Could you check a few things on this model? Use its own coordinates, in mm. A direction names the side the tool comes from. Give positions to 0.01 mm unless a question says otherwise; leave off trailing zeros. Write item = value, one per line.
from build123d import *

# Parameters (mm, degrees)
F0_W     = 12.5
F0_H     = 2.5
F2_W     = 5
F2_H     = 30
F3_DEPTH = 6


# Not quite as in the source:
# - a fillet or chamfer that OpenCascade refuses, or shapes differently, is made with other operations: its cross-section is extruded or revolved along the edge and cut away or added


with BuildPart() as f1:
    # F0 (on Front) → F1 (revolve)
    with BuildSketch(Plane.XZ):
        with BuildLine():
            Line((0, 2.5), (12.5, 2.5))
            add(Edge.make_bspline(
                [(8, 38), (7.0575290046, 36.0296102259), (4.9176459622, 31.9169764445), (8.8571855748, 23.8819266131), (11.7311727266, 17.2522437772), (5.0634432181, 9.5532988579), (9.6973287885, 5.0417102196), (12.5, 2.5)],
                knots=[0, 0, 0, 0, 0.1821407595, 0.3923850866, 0.5803644457, 0.7831417696, 1, 1, 1, 1], degree=3))
            Line((8, 38), (0, 38))
            Line((0, 38), (0, 2.5))
        make_face()
        with Locations((6.25, 1.25)):
            Rectangle(F0_W, F0_H)
        Polygon((10, 40), (10, 48), (8, 48), (8, 40), (0, 40), (0, 38), (8, 38), align=None)
    revolve(axis=Axis((0, 0, 44), (0, 0, -1)))

    # F2 (on face) → F3 (cut)
    with BuildSketch(Plane.XY.offset(48)):
        Rectangle(F2_W, F2_H)
    extrude(amount=-F3_DEPTH, mode=Mode.SUBTRACT)

    # F4: chamfer of 5 on 1 edges, made by hand


with BuildPart() as f4_tool2:
    # F4_s3 → F4_t4 (revolve)
    with BuildSketch(Plane.XZ):
        Polygon((8, 45), (3, 40), (8, 40), align=None)
    revolve(axis=Axis((0, 0, 40), (0, 0, -1)))

    split(bisect_by=Plane.YZ.offset(2.5), keep=Keep.TOP)


with BuildPart() as f1_1:
    add(f1.part)

    # F4_t1: union F4_tool2
    add(f4_tool2.part)


with BuildPart() as f4_tool7:
    # F4_s8 → F4_t9 (revolve)
    with BuildSketch(Plane.XZ):
        Polygon((8, 45), (3, 40), (8, 40), align=None)
    revolve(axis=Axis((0, 0, 40), (0, 0, -1)))

    split(bisect_by=Plane.XY.offset(42), keep=Keep.BOTTOM)


with BuildPart() as f1_2:
    add(f1_1.part)

    # F4_t6: union F4_tool7
    add(f4_tool7.part)


with BuildPart() as f4_tool12:
    # F4_s13 → F4_t14 (revolve)
    with BuildSketch(Plane.XZ):
        Polygon((8, 45), (3, 40), (8, 40), align=None)
    revolve(axis=Axis((0, 0, 40), (0, 0, -1)))

    split(bisect_by=Plane.YZ.offset(-2.5), keep=Keep.BOTTOM)


with BuildPart() as f1_3:
    add(f1_2.part)

    # F4_t11: union F4_tool12
    add(f4_tool12.part)


solid = f1_3.part
1. Thinking about a two-plate mould opening in Y: for faces 5 (the face through (0, -7, 42)), 6 (the face through (8, 0, 46)), 7 (the face through (11.923, -3.755, 1.268)), which applies, pulls with the +Y half, pulls with the -Y half, needs draft (parallel to the pull), parting line crosses it, or undercut?
Filled sheet:
face_5 = needs draft
face_6 = undercut
face_7 = parting line crosses it
2. For pin 1 (6 mm diameter, centred on y = 7, z = 44, fed in from +X); pin 2 (2.5 mm diameter, centred on x = 1, y = 7.5, fed in from +Z); pin 3 (1.6 mm diameter, centred on y = 8.5, z = 46, fed in from -X), each with a flat end and sliding along its axis, tell me the tip position at first contact or that it passes through.
Filled sheet:
pin_1 = 9.17
pin_2 = 42
pin_3 = -6.38
3. Which directions (+Z, -Z, +X, -X, +Y, -Y) give clear straight access to the entire face, cutting with the end or side of a thin tool? Please do faces 1 (the face through (2.5, -8, 44)), 2 (the face through (-8, 0, 46)), 3 (the face through (-1.06, -8.06, 38.13)), 4 (the face through (-8.2, 0, 48)).
Filled sheet:
face_1 = +Z, +Y, -Y
face_2 = +Z
face_3 = none
face_4 = +Z, +X, -X, +Y, -Y
4. I need wall thicknesses on line 1 (Z direction, x = 4.5, y = -7.5); line 2 (Z direction, x = -8.5, y = -4.5); line 3 (Z direction, x = -4.75, y = 5.5). Which ranges of each line are inside material? Lowest first, please.
Filled sheet:
line_1 = 0 to 6.36, 13.84 to 23.97, 38.75 to 48
line_2 = 0 to 5.3, 15.57 to 21.99, 39.62 to 48
line_3 = 0 to 27.28, 36.46 to 44.27
